For this review, use the dimensioned drawing (mm, ordinates from the lowest corner) and the shaded views. Coordinates: 2 decimals unless noted, no trailing zeros. Loops run counter-clockwise (first coordinate to the right, second up) from the corner with the lowest first, then second, coordinate; pieces in that order, holes last. Notation, with made-up numbers: M 76,13.25 L 131,13.25 A28 cw 131,40.25 Z; hole C -4,87 d10. An arc over 180 degrees is marked long. Write item = value, one per line. Start each with the question number.
Q1. Clearance check with flat-ended pins moving along their axes: pin 1 Ø8 at (x, z) = (772, 413.5) entering from +Y; pin 2 Ø4 at (x, z) = (437, 356) entering from -Y; pin 3 Ø1.5 at (x, z) = (599, 154.5) entering from -Y. State where each tip first meets the part, or that it passes through.
Q2. We need section A-A on z = 277.5. Give the boundary of the cut face in (x, y), and give its area (3 significant figures).
Q3. We need section B-B on y = 475. Give the boundary of the cut face in (x, z).
Q4. Mouldability with a two-part tool opening along Y and no side actions: class the marked faces 1, 2 and 3 as released by +Y, released by -Y, zero draft, split by the parting line, or undercut.
Q5. We need section C-C on y = 260. Give the boundary of the cut face in (x, z), and give its area (3 significant figures).
Q6. Wall thickness on probe 1 along Y at (x, z) = (469.5, 474); probe 2 along X at (y, z) = (334.5, 391.5); probe 3 along X at (y, z) = (712, 537): over which ranges is each line inside the solid? List them lowest first.
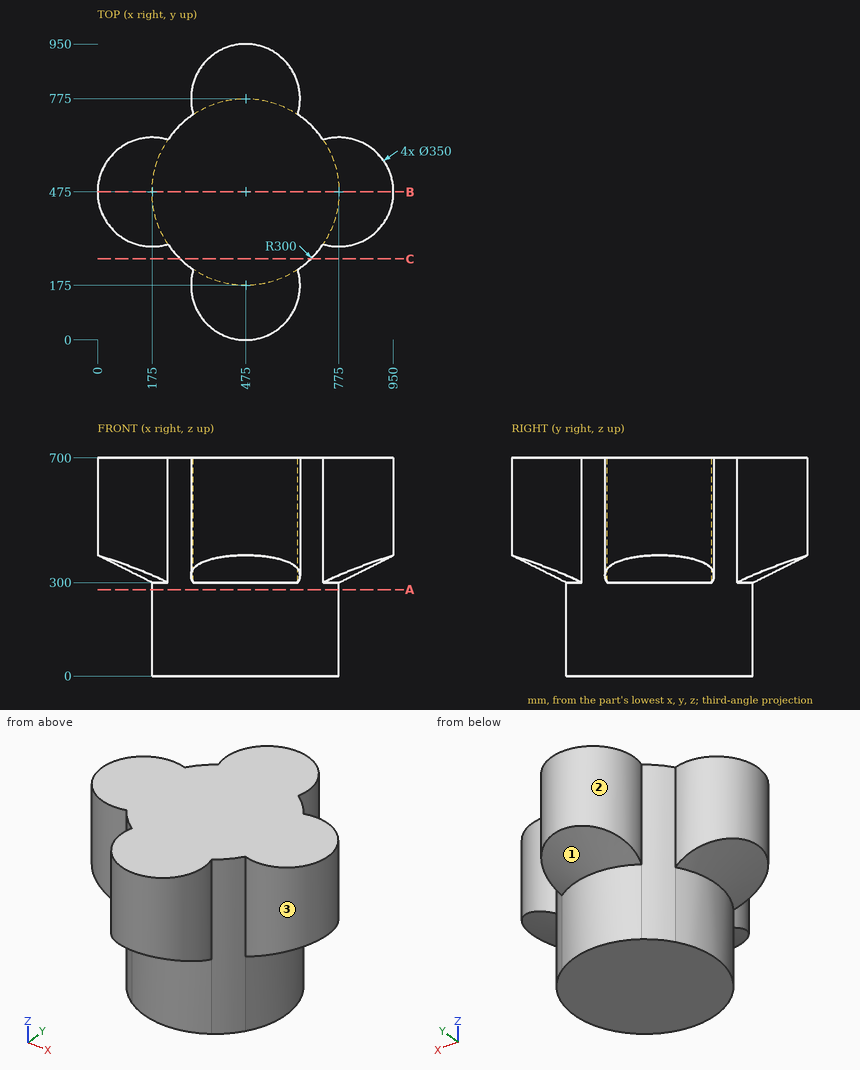
Returned:
q1.pin_1 = 650
q1.pin_2 = 60.74
q1.pin_3 = 201.49
q2.outline = C 475,475 d600
q2.area = 283,000 mm^2
q3.outline = M 0,387.5 L 175,300 L 175,0 L 775,0 L 775,300 L 950,387.5 L 950,700 L 0,700 Z
q4.face_1 = released by +Y
q4.face_2 = undercut
q4.face_3 = split by the parting line
q5.outline = M 265.78,0 L 684.22,0 L 684.22,700 L 265.78,700 Z
q5.area = 293,000 mm^2
q6.probe_1 = 0.09 to 949.91
q6.probe_2 = 70.67 to 879.33
q6.probe_3 = 291.07 to 658.93
